```python
from build123d import *

# Parameters (mm, degrees)
SKETCH2_R            = 6.985
BOSS_EXTRUDE11_DEPTH = 116.84
SKETCH2_4_R          = 6.985
BOSS_EXTRUDE12_DEPTH = 63.5
SKETCH19_W           = 13.97
SKETCH19_H           = 50.8
BOSS_EXTRUDE13_DEPTH = 15.24
SKETCH21_R           = 6.985
BOSS_EXTRUDE15_DEPTH = 15.24


with BuildPart() as part:
    # Sketch2 → Boss-Extrude11 (new body)
    with BuildSketch(Plane.XY):
        with Locations(Location((0, 0, 0), (0, 0, 180))):
            Circle(SKETCH2_R)
    extrude(amount=BOSS_EXTRUDE11_DEPTH)



with BuildPart() as body_2:
    # Sketch2_4 → Boss-Extrude12 (new body)
    with BuildSketch(Plane.XY):
        with Locations((0, -50.8)):
            Circle(SKETCH2_4_R)
    extrude(amount=BOSS_EXTRUDE12_DEPTH)


with BuildPart() as part_1:
    add(part.part)

    add(body_2.part)  # Boss-Extrude13 merges body 2
    # Sketch19 → Boss-Extrude13 (add)
    with BuildSketch(Plane.XY.offset(63.5)):
        with Locations((0, -25.4)):
            Rectangle(SKETCH19_W, SKETCH19_H)
    extrude(amount=BOSS_EXTRUDE13_DEPTH)

    # Sketch21 → Boss-Extrude15 (add)
    with BuildSketch(Plane.XY.offset(63.5)):
        with Locations((0, -50.8)):
            Circle(SKETCH21_R)
    extrude(amount=BOSS_EXTRUDE15_DEPTH)


solid = part_1.part
```
Check sheet for the modelled part. Datum: model origin and axes. Units: mm. A direction names the side the tool comes from. Round coordinates to 2 decimals unless told otherwise and drop trailing zeros. Loops run counter-clockwise (first coordinate to the right, second up) from the corner with the lowest first, then second, coordinate; pieces in that order, holes last. Notation, with made-up numbers: (-4, 25.25) - (13, 25.25) arc R17 cw to (13, 50.25) - close; hole circle Ø3 at (64.25, 40). An arc over 180 degrees is marked (long way). Write item = value, one per line. Start each with the question number.
Q1. Depth check by flat-ended pin: P1, Ø2, axis at x = -5, z = 57, coming from the -Y side; P2, Ø5, axis at x = 0, y = -27, coming from the -Z side; P3, Ø7, axis at x = 0, y = -32.5, coming from the +Z side. Enter the tip coordinate at first touch or a pass-through.
Q2. Section check C-C (y = -19.5). Record the boundary of the cut face in (x, z) (3 decimals), plus the area to 3 significant figures.
Q3. Section check B-B (x = 0). Record the boundary of the cut face in (y, z) (3 decimals), plus the area to 3 significant figures.
Q4. Thickness scan on L1, parallel to Z at x = -0.25, y = -37.5; L2, parallel to Y at x = -2.75, z = 46.5; L3, parallel to Y at x = 2.25, z = 8. Record the ranges inside material, lowest first.
Q5. Release check for a two-part mould opening along Y. For faces 1 (the face through (0, 0, 0)), 2 (the face through (-3.22, 6.2, 57.6)) record: pulls with the +Y half, pulls with the -Y half, needs draft (parallel to the pull), parting line crosses it, or undercut.
Q6. Access from +Z, -Z, +X, -X, +Y, -Y to the whole of each face (thin tool, end or side, straight path). Record for faces 3 (the face through (-1.51, -57.62, 38.82)), 4 (the face through (0, -51, 0)).
Q7. Section check D-D (x = 5). Record the boundary of the cut face in (y, z).
Q8. Section check A-A (z = 33.5). Record the boundary of the cut face in (x, y) (3 decimals), plus the area to 3 significant figures.
Derived:
q1.P1 = -56.53
q1.P2 = 63.5
q1.P3 = 78.74
q2.outline = (-6.985, 63.5) - (6.985, 63.5) - (6.985, 78.74) - (-6.985, 78.74) - close
q2.area = 213 mm^2
q3.outline = (-57.785, 0) - (-43.815, 0) - (-43.815, 63.5) - (-6.985, 63.5) - (-6.985, 0) - (6.985, 0) - (6.985, 116.84) - (-6.985, 116.84) - (-6.985, 78.74) - (-57.785, 78.74) - close
q3.area = 3,290 mm^2
q4.L1 = 63.5 to 78.74
q4.L2 = -57.22 to -44.38, -6.42 to 6.42
q4.L3 = -57.41 to -44.19, -6.61 to 6.61
q5.face_1 = needs draft
q5.face_2 = undercut
q6.face_3 = -Z
q6.face_4 = -Z, +X, -X, +Y, -Y
q7.outline = (-55.68, 0) - (-45.92, 0) - (-45.92, 63.5) - (-4.88, 63.5) - (-4.88, 0) - (4.88, 0) - (4.88, 116.84) - (-4.88, 116.84) - (-4.88, 78.74) - (-55.68, 78.74) - close
q8.outline = circle Ø13.97 at (0, -50.8); circle Ø13.97 at (0, 0)
q8.area = 307 mm^2
